Work out the finished part from the listing and answer in its coordinate system (mm). Face numbers are marked on the shaded views. A direction names the side the tool comes from. Give positions to 0.01 mm unless a question says otherwise; leave off trailing zeros. Loops run counter-clockwise (first coordinate to the right, second up) from the corner with the lowest first, then second, coordinate; pieces in that order, holes last. Notation, with made-up numbers: (50, -6.75) - (70, -6.75) arc R28 cw to (70, 27.25) - close; hole circle Ø3 at (58.5, 34.25). An arc over 180 degrees is marked (long way). One line per item, written item: value.
from build123d import *

# Parameters (mm, degrees)
SKETCH1_W           = 23
SKETCH1_H           = 15
BOSS_EXTRUDE1_DEPTH = 3
SKETCH10_W          = 3
SKETCH10_H          = 15
BOSS_EXTRUDE2_DEPTH = 20
SKETCH13_R          = 1.75
CUT_EXTRUDE3_DEPTH  = 24
SKETCH14_R          = 1.75
CUT_EXTRUDE4_DEPTH  = 24
FILLET1_R           = 3
SKETCH15_W          = 3
SKETCH15_H          = 15
BOSS_EXTRUDE3_DEPTH = 10
SKETCH16_W          = 13
SKETCH16_H          = 15
BOSS_EXTRUDE4_DEPTH = 10
SKETCH17_R          = 1.75
CUT_EXTRUDE5_DEPTH  = 16


with BuildPart() as part:
    # Sketch1 → Boss-Extrude1 (new body)
    with BuildSketch(Plane.XY):
        Rectangle(SKETCH1_W, SKETCH1_H)
    extrude(amount=BOSS_EXTRUDE1_DEPTH)

    # Sketch10 → Boss-Extrude2 (add)
    with BuildSketch(Plane.XY.offset(3)):
        with Locations((-10, 0)):
            Rectangle(SKETCH10_W, SKETCH10_H)
    extrude(amount=BOSS_EXTRUDE2_DEPTH)

    # Sketch13 → Cut-Extrude3 (cut, through all)
    with BuildSketch(Plane(origin=(0, 0, 0), x_dir=(-1, 0, 0), z_dir=(0, 0, -1))):
        with Locations((-3.5, 0)):
            Circle(SKETCH13_R)
    extrude(amount=-CUT_EXTRUDE3_DEPTH, mode=Mode.SUBTRACT)

    # Sketch14 → Cut-Extrude4 (cut, through all)
    with BuildSketch(Plane.ZY.offset(11.5)):
        with Locations((15, 0)):
            Circle(SKETCH14_R)
    extrude(amount=-CUT_EXTRUDE4_DEPTH, mode=Mode.SUBTRACT)

    # Fillet1
    fillet1_edges = [part.edges().sort_by_distance(p)[0] for p in [
        (-11.5, 0, 0),
    ]]
    fillet(fillet1_edges, radius=FILLET1_R)

    # Sketch15 → Boss-Extrude3 (add)
    with BuildSketch(Plane.XY.offset(23)):
        with Locations((-10, 0)):
            Rectangle(SKETCH15_W, SKETCH15_H)
    extrude(amount=BOSS_EXTRUDE3_DEPTH)

    # Sketch16 → Boss-Extrude4 (add)
    with BuildSketch(Plane.ZY.offset(11.5)):
        with Locations((26.5, 0)):
            Rectangle(SKETCH16_W, SKETCH16_H)
    extrude(amount=BOSS_EXTRUDE4_DEPTH)

    # Sketch17 → Cut-Extrude5 (cut, through all)
    with BuildSketch(Plane.XZ.offset(7.5)):
        with Locations((-15, 26.5)):
            Circle(SKETCH17_R)
    extrude(amount=-CUT_EXTRUDE5_DEPTH, mode=Mode.SUBTRACT)


solid = part.part
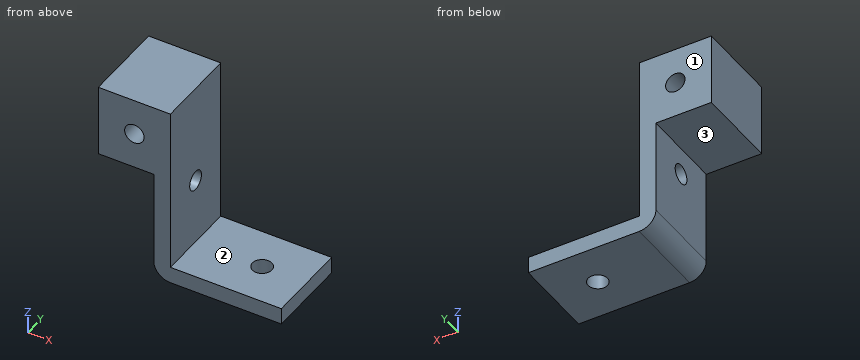
1. Section C-C (z = 26.5) is taken. Write down the section's boundary in (x, y), and give its area (4 significant figures).
Output:
outline: (-21.5, -7.5) - (-16.75, -7.5) - (-16.75, 7.5) - (-21.5, 7.5) - close; (-13.25, -7.5) - (-8.5, -7.5) - (-8.5, 7.5) - (-13.25, 7.5) - close
area: 142.5 mm²
2. Section B-B (x = -15) is taken. Write down the section's boundary in (y, z).
Output:
outline: (-7.5, 20) - (7.5, 20) - (7.5, 24.75) - (-7.5, 24.75) - close; (-7.5, 28.25) - (7.5, 28.25) - (7.5, 33) - (-7.5, 33) - close
3. Section D-D (y = -3.75) is taken. Write down the section's boundary in (x, z), and give its area (3 significant figures).
Output:
outline: (-21.5, 20) - (-11.5, 20) - (-11.5, 3) arc R3 ccw to (-8.5, 0) - (11.5, 0) - (11.5, 3) - (-8.5, 3) - (-8.5, 33) - (-21.5, 33) - close; hole circle Ø3.5 at (-15, 26.5)
area: 277 mm²
4. Section A-A (y = 0) is taken. Write down the section's boundary in (x, z).
Output:
outline: (-21.5, 20) - (-11.5, 20) - (-11.5, 16.75) - (-8.5, 16.75) - (-8.5, 33) - (-21.5, 33) - close; (-11.5, 3) arc R3 ccw to (-8.5, 0) - (1.75, 0) - (1.75, 3) - (-8.5, 3) - (-8.5, 13.25) - (-11.5, 13.25) - close; (5.25, 0) - (11.5, 0) - (11.5, 3) - (5.25, 3) - close; hole circle Ø3.5 at (-15, 26.5)
5. Find the intervals of material crossed by line 1 along Y through (x, z) = (-10.1, 15); line 2 along X through (y, z) = (-0.5, 10); line 3 along Z through (x, y) = (-2, -0.5), in increasing order.
Output:
line 1: y = -7.5 to -1.75, 1.75 to 7.5
line 2: x = -11.5 to -8.5
line 3: z = 0 to 3
6. Flat-ended cylindrical pins translate along their axes: pin 1 Ø8 at (x, z) = (-14.5, 26.5) entering from -Y; pin 2 Ø1.5 at (x, y) = (-7, 5.5) entering from +Z; pin 3 Ø4 at (y, z) = (0, 15) entering from -X; pin 4 Ø5 at (x, y) = (-17, 1.5) entering from -Z. Find the tip coordinate at first contact, or state that the pin passes through.
Output:
pin 1: stops at y = -7.5
pin 2: stops at z = 3
pin 3: stops at x = -11.5
pin 4: stops at z = 20
7. For the marked faces 1, 2 and 3, determine the directions among +Z, -Z, +X, -X, +Y, -Y from which every point of the face is accessible in a straight line to the end or side of a thin tool.
Output:
face 1: +Z, -Z, +X, -X, +Y
face 2: +Z, +X, +Y, -Y
face 3: -Z, -X, +Y, -Y
